For this review, take the finished solid that the model builds, in its own axes (mm). A direction names the side the tool comes from. Round coordinates to 2 decimals unless told otherwise and drop trailing zeros. One line per question, with ' | ' between items. Start each with the question number.
1. Draft analysis for pull direction Y (two halves, no side actions). For faces 1 (the face through (8.63, -16.59, 0.15)), 2 (the face through (0, -4.5, 1)), 3 (the face through (0, 0, 0)), state which applies: pulls with the +Y half, pulls with the -Y half, needs draft (parallel to the pull), parting line crosses it, or undercut.
2. Wall thickness on line 1 along Z through (x, y) = (-15.5, -6); line 2 along Z through (x, y) = (-14, -2); line 3 along Z through (x, y) = (-1.5, -9.5): over which ranges is each line inside the solid? List them lowest first.
3. For faces 4 (the face through (-4, 0, 2.3)), 5 (the face through (-4.5, 0, 1)), list the 3-axis set-ups (+Z, -Z, +X, -X, +Y, -Y) from which the entire face can be reached by the end or side of a thin tool; tool diameter is ignored.
4. For pin 1 Ø1 at (y, z) = (6.5, 1) entering from +X; pin 2 Ø0.8 at (y, z) = (-0.5, 1.5) entering from -X; pin 3 Ø0.5 at (y, z) = (0.5, 1.5) entering from +X; pin 4 Ø5 at (x, y) = (2.5, -11) entering from -Z, all flat-tipped, find the tip position at first contact; note any pin that passes through.
```python
from build123d import *

# Parameters (mm, degrees)
F0_R      = 18.7
F0_R_2    = 13.7
F1_DEPTH  = 0.3
F2_DEPTH  = 2
F2_TAPER  = -24
F4_R      = 0.6
F8_W      = 9
F8_H      = 9
F9_DEPTH  = 2
F10_R     = 0.5
F11_W     = 6.4
F11_H     = 6.4
F12_DEPTH = 2
F13_R     = 1.5


# Not quite as in the source:
# - a fillet or chamfer that OpenCascade refuses, or shapes differently, is made with other operations: its cross-section is extruded or revolved along the edge and cut away or added


with BuildPart() as f1:
    # F0 (on Top) → F1 (new body)
    with BuildSketch(Plane.XY):
        Circle(F0_R)
        Circle(F0_R_2, mode=Mode.SUBTRACT)
        Circle(F0_R_2)
    extrude(amount=F1_DEPTH)

    # F0 (on Top) → F2 (join)
    with BuildSketch(Plane.XY):
        Circle(F0_R_2)
    extrude(amount=F2_DEPTH, taper=F2_TAPER)

    # F3: chamfer of 0.6 on 1 edges, made by hand

    # F3_s1 → F3_t2 (revolve, cut)
    with BuildSketch(Plane.XZ):
        Polygon((14.3464153848, 1.4518727254), (13.9904573706, 2), (14.5904573706, 2), align=None)
    revolve(axis=Axis((0, 0, 2), (0, 0, -1)), mode=Mode.SUBTRACT)

    # F4
    f4_edges = [f1.edges().sort_by_distance(p)[0] for p in [
        (-14.346415, 0, 1.451873),
        (-13.990457, 0, 2),
    ]]
    fillet(f4_edges, radius=F4_R)


with BuildPart() as f6:
    # F5 (on Front) → F6 (revolve)
    with BuildSketch(Plane.XZ):
        with BuildLine():
            Line((0, 2), (-13.6646839508, 2))
            add(Edge.make_bspline(
                [(-13.6646839508, 2), (-11.1315483197, 2), (-12.2314980254, 0.6), (0, 0.6)],
                knots=[0, 0, 0, 0, 13.7362144522, 13.7362144522, 13.7362144522, 13.7362144522], degree=3))
            Line((0, 0.6), (0, 2))
        make_face()
    revolve(axis=Axis((0, 0, 1.3), (0, 0, -1)))


with BuildPart() as f1_1:
    add(f1.part)

    # F7: cut F6
    add(f6.part, mode=Mode.SUBTRACT)

    # F8 (on face) → F9 (join)
    with BuildSketch(Plane.XY.offset(0.3)):
        Rectangle(F8_W, F8_H)
    extrude(amount=F9_DEPTH)

    # F10
    f10_edges = [f1_1.edges().sort_by_distance(p)[0] for p in [
        (-4.5, 4.5, 1.538289),
        (-4.5, -4.5, 1.538289),
        (4.5, -4.5, 1.538289),
        (4.5, 4.5, 1.538289),
    ]]
    fillet(f10_edges, radius=F10_R)

    # F11 (on face) → F12 (cut, through all)
    with BuildSketch(Plane.XY.offset(2.3)):
        Rectangle(F11_W, F11_H)
    extrude(amount=-F12_DEPTH, mode=Mode.SUBTRACT)

    # F13
    f13_edges = [f1_1.edges().sort_by_distance(p)[0] for p in [
        (-3.2, 3.2, 1.3),
        (3.2, 3.2, 1.3),
        (3.2, -3.2, 1.3),
        (-3.2, -3.2, 1.3),
        (0, -3.2, 0.3),
        (3.2, 0, 0.3),
        (0, 3.2, 0.3),
        (-3.2, 0, 0.3),
    ]]
    fillet(f13_edges, radius=F13_R)


solid = f1_1.part
```
Answer block:
1) face 1: parting line crosses it | face 2: undercut | face 3: needs draft
2) line 1: z = 0 to 0.3 | line 2: z = 0 to 0.3, 0.99 to 1.76 | line 3: z = 0 to 1.13
3) face 4: +Z, +X, -X, +Y, -Y | face 5: +Z
4) pin 1: stops at x = 12.89 | pin 2: stops at x = -14.27 | pin 3: stops at x = 14.26 | pin 4: stops at z = 0
